CAD build for the part. Positions are in the model's coordinates, mm. A direction names the side the tool comes from. Round coordinates to 2 decimals unless told otherwise and drop trailing zeros. Order: outer loops, then holes, each group sorted by start corner. A loop starts at its lowest first (then second) coordinate and runs counter-clockwise, first axis right, second up. Notation, with made-up numbers: M -30.75,-36.75 L 24.25,-36.75 A13 cw 24.25,-26.75 Z; hole C 63,11 d10. An arc over 180 degrees is marked long. Answer as a JSON object with one key per item and string values.
```python
from build123d import *

# Parameters (mm, degrees)
F0_W      = 38.1
F0_H      = 25.4
F1_DEPTH  = 25.4
F3_DEPTH  = 25.401
F4_W      = 11.4385973006
F4_H      = 17.5851260588
F5_DEPTH  = 12.7
F7_DEPTH  = 12.7
F9_DEPTH  = 25.4
F10_W     = 12.7
F10_H     = 2.1544784386
F11_DEPTH = 0.254


with BuildPart() as f1:
    # F0 (on Front) → F1 (new body)
    with BuildSketch(Plane.XZ):
        with Locations((19.05, 12.7)):
            Rectangle(F0_W, F0_H)
    extrude(amount=F1_DEPTH)

    # F2 (on face) → F3 (cut, through all)
    with BuildSketch(Plane.XZ.offset(25.4)):
        Polygon((38.1, 25.4), (27.6416484267, 25.4), (38.1, 9.3479026109), align=None)
    extrude(amount=-F3_DEPTH, mode=Mode.SUBTRACT)

    # F4 (on face) → F5 (cut)
    with BuildSketch(Plane(origin=(0, 0, 0), x_dir=(0, -1, 0), z_dir=(-1, 0, 0))):
        with Locations((19.6807013497, 16.6074369706)):
            Rectangle(F4_W, F4_H)
    extrude(amount=-F5_DEPTH, mode=Mode.SUBTRACT)

    # F6 (on face) → F7 (cut)
    with BuildSketch(Plane.XZ.offset(25.4)):
        Polygon((22.0128018409, 25.4), (22.0128018409, 7.8148739412), (38.1, 7.8148739412), (38.1, 9.3479026109), (27.6416484267, 25.4), align=None)
    extrude(amount=-F7_DEPTH, mode=Mode.SUBTRACT)

    # F8 (on face) → F9 (cut)
    with BuildSketch(Plane.YZ.offset(22.0128018409)):
        Polygon((-25.4, 25.4), (-25.4, 7.8148739412), (-12.7, 25.4), align=None)
    extrude(amount=-F9_DEPTH, mode=Mode.SUBTRACT)

    # F10 (on face) → F11 (cut)
    with BuildSketch(Plane(origin=(0, -20.4024901747, 14.7347038828), x_dir=(1, 0, 0), z_dir=(0, -0.8106872987, 0.5854793795))):
        with Locations((6.35, 12.0786300472)):
            Rectangle(F10_W, F10_H)
    extrude(amount=-F11_DEPTH, mode=Mode.SUBTRACT)


solid = f1.part
```
Item 1: 3-axis set-ups, long thin cutter, end or side, ignore diameter. For faces 1 (the flat face through (30, -19, 7.815)), 2 (the flat face through (6, -13.961, 16)), 3 (the flat face through (38.1, -13, 5)): which of +Z, -Z, +X, -X, +Y, -Y reach the whole face in a straight line?
Worked answers:
{"face 1": "+Z, +X, -Y", "face 2": "+Z, -X, -Y", "face 3": "+Z, -Z, +X, +Y, -Y"}
Item 2: Saw through at B-B on x = 25. List the corners of the cut face in (y, z), and give its area (3 significant figures).
Worked answers:
{"outline": "M -25.4,0 L 0,0 L 0,25.4 L -12.7,25.4 L -12.7,7.81 L -25.4,7.81 Z", "area": "422 mm2"}
Item 3: Drop flat-ended pins along their axis: pin 1 Ø3.5 at (y, z) = (-17, 17.5) entering from -X; pin 2 Ø2 at (x, y) = (12.5, -20) entering from +Z; pin 3 Ø9 at (x, y) = (7, -20.5) entering from +Z. Give the stop position or say it passes through.
Worked answers:
{"pin 1": "stops at x = 12.7", "pin 2": "stops at z = 16.65", "pin 3": "stops at z = 7.81"}
Item 4: Saw through at D-D on x = 16. List the corners of the cut face in (y, z).
Worked answers:
{"outline": "M -25.4,0 L 0,0 L 0,25.4 L -12.7,25.4 L -25.4,7.81 Z"}
Item 5: Saw through at C-C on z = 22. List the corners of the cut face in (x, y).
Worked answers:
{"outline": "M 0,-13.96 L 12.7,-13.96 L 12.7,-15.16 L 22.01,-15.16 L 22.01,-12.7 L 29.86,-12.7 L 29.86,0 L 0,0 Z"}
Item 6: Wall check: line 1 along Z through (x, y) = (33.5, -14.75); line 2 along Y through (x, z) = (9, 21.75); line 3 along Y through (x, z) = (35, 12.25). Give the ranges that are in metal, low to high. Write a range as [from, to].
Worked answers:
{"line 1": "z = [0, 7.81]", "line 2": "y = [-13.96, 0]", "line 3": "y = [-12.7, 0]"}
Item 7: Saw through at A-A on y = -11.75. List the corners of the cut face in (x, z).
Worked answers:
{"outline": "M 0,0 L 38.1,0 L 38.1,9.35 L 27.64,25.4 L 0,25.4 Z"}
